from build123d import *

# Parameters (mm, degrees)
SKETCH_W     = 60
SKETCH_H     = 100
PAD_DEPTH    = 5
SKETCH001_R  = 2.1
PAD001_DEPTH = 1
SKETCH002_W  = 5
SKETCH002_H  = 35.7
PAD002_DEPTH = 1
FILLET_R     = 10
FILLET001_R  = 10
FILLET002_R  = 10


with BuildPart() as part:
    # Sketch → Pad (new body)
    with BuildSketch(Plane.XY):
        Rectangle(SKETCH_W, SKETCH_H)
    extrude(amount=PAD_DEPTH)

    # Sketch001 (on DatumPlane) → Pad001 (join, symmetric)
    with BuildSketch(Plane.XZ.offset(25)):
        with BuildLine():
            Line((-5, 52), (-5, 5))
            Line((-5, 5), (-15, 5))
            Line((-15, 5), (-15, 52))
            ThreePointArc((-5, 52), (-10, 57), (-15, 52))
        make_face()
        with Locations((-10, 50)):
            Circle(SKETCH001_R, mode=Mode.SUBTRACT)
        with Locations((-10, 40)):
            Circle(SKETCH001_R, mode=Mode.SUBTRACT)
    extrude(amount=PAD001_DEPTH, both=True)

    # Sketch002 (on DatumPlane) → Pad002 (join, symmetric)
    with BuildSketch(Plane.XZ.offset(-25)):
        with Locations((0, 22.85)):
            Rectangle(SKETCH002_W, SKETCH002_H)
    extrude(amount=PAD002_DEPTH, both=True)

    # Sketch003 (on DatumPlane) → Revolution (revolve)
    with BuildSketch(Plane.XZ.offset(-25)):
        with BuildLine():
            ThreePointArc((2.731847, 48.255689), (0, 49.25), (-2.731847, 48.255689))
            Line((-2.731847, 49.483248), (-2.731847, 48.255689))
            ThreePointArc((2.731847, 49.483248), (0, 50.25), (-2.731847, 49.483248))
            Line((2.731847, 48.255689), (2.731847, 49.483248))
        make_face()
    revolve(axis=Axis((0, 25, 45), (1, 0, 0)))

    # Fillet
    fillet_edges = [part.edges().sort_by_distance(p)[0] for p in [
        (-10, -26, 5),
        (-10, -24, 5),
    ]]
    fillet(fillet_edges, radius=FILLET_R)

    # Fillet001
    fillet001_edges = [part.edges().sort_by_distance(p)[0] for p in [
        (0, 24, 5),
        (0, 26, 5),
    ]]
    fillet(fillet001_edges, radius=FILLET001_R)

    # Fillet002
    fillet002_edges = [part.edges().sort_by_distance(p)[0] for p in [
        (-30, -50, 2.5),
        (-30, 50, 2.5),
        (30, 50, 2.5),
        (30, -50, 2.5),
    ]]
    fillet(fillet002_edges, radius=FILLET002_R)


solid = part.part
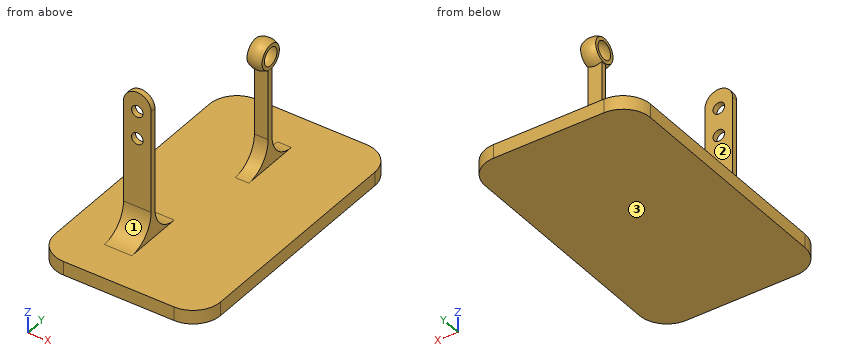
Build history of the part. All positions in model axes, mm. Face numbers are marked on the shaded views. Round coordinates to 2 decimals unless told otherwise and drop trailing zeros. Order: outer loops, then holes, each group sorted by start corner. A loop starts at its lowest first (then second) coordinate and runs counter-clockwise, first axis right, second up. Notation, with made-up numbers: M 58.25,60 L 62.25,60 A29 ccw 62.25,97 Z; hole C 43.25,30 d4. An arc over 180 degrees is marked long. Use CSV: the item, a comma, the result in double quotes. Start each with the question number.
(1) Cut at D-D on x = 14.5. List the corners of the cut face in (y, z).
(2) Drill centre lines: probe 1 along Z at (x, y) = (-10, -25.05); probe 2 along Z at (x, y) = (1, -13); probe 3 along Y at (x, z) = (-6, 37). Where is each one in solid material? Low to high.
(3) Cut at B-B on x = -10. List the corners of the cut face in (y, z).
(4) Cut at C-C on y = 4.5. List the corners of the cut face in (x, z), then the cut area to 3 significant figures.
(5) Cut at A-A on z = 18.5. List the corners of the cut face in (x, y), then the cut area to 3 significant figures.
(6) Mould opens along Z. For the marked faces 1, 2 and 3 say: +Z half, -Z half, draft (parallel to the pull), parting line (faces both ways), or undercut.
(7) Flat gauge pins, fed straight in: P1, Ø7, axis at y = 24, z = 44, coming from the +X side; P2, Ø1.5, axis at x = -1, z = 22.5, coming from the -Y side; P3, Ø2.5, axis at y = 23, z = 43.5, coming from the -X side. Where does each tip first touch, or does it go through?
Findings:
1,outline,"M -50,0 L 50,0 L 50,5 L -50,5 Z"
2,probe 1,"z = 0 to 37.9, 42.1 to 47.9, 52.1 to 57"
2,probe 2,"z = 0 to 5"
2,probe 3,"y = -26 to -24"
3,outline,"M -50,0 L 50,0 L 50,5 L -14,5 A10 cw -24,15 L -24,37.9 L -26,37.9 L -26,15 A10 cw -36,5 L -50,5 Z; M -26,42.1 L -24,42.1 L -24,47.9 L -26,47.9 Z; M -26,52.1 L -24,52.1 L -24,57 L -26,57 Z"
4,outline,"M -30,0 L 30,0 L 30,5 L -30,5 Z"
4,area,"300 mm^2"
5,outline,"M -15,-26 L -5,-26 L -5,-24 L -15,-24 Z; M -2.5,24 L 2.5,24 L 2.5,26 L -2.5,26 Z"
5,area,"30.0 mm^2"
6,face 1,"+Z half"
6,face 2,"draft"
6,face 3,"-Z half"
7,P1,"stops at x = 2.73"
7,P2,"stops at y = 24"
7,P3,"stops at x = -2.73"
